Answer from the drawing. Dimensions are ordinates in mm from the lowest x, y and z of the part. Give positions to 0.01 mm unless a question says otherwise; leave off trailing zeros. Order: outer loops, then holes, each group sorted by start corner. A loop starts at its lowest first (then second) coordinate and runs counter-clockwise, first axis right, second up. Notation, with made-up numbers: (69.25, 32) - (115.25, 32) arc R19 ccw to (115.25, 69) - close; hole circle Ø4 at (37.5, 69.5). An arc over 180 degrees is marked (long way). Write each question's results on one line, items separated by ' | '.
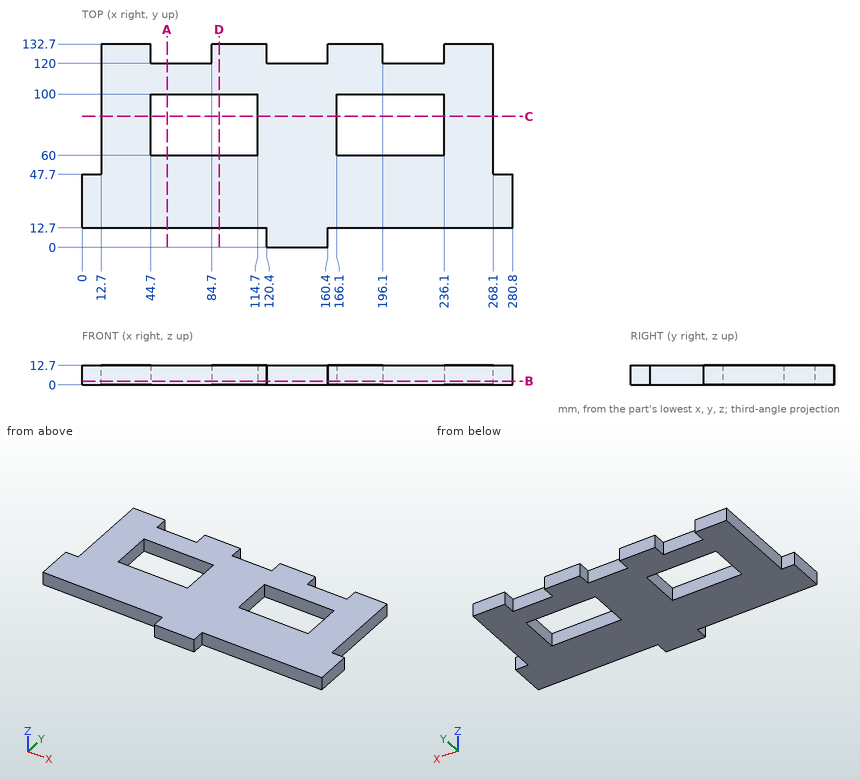
(1) Section A-A (x = 55.5) is taken. Give the vertices of the cut face in (y, z).
Conclusion:
outline: (12.7, 0) - (60, 0) - (60, 12.7) - (12.7, 12.7) - close; (100, 0) - (120, 0) - (120, 12.7) - (100, 12.7) - close
(2) Section B-B (z = 2.5) is taken. State how many separate pieces and enclosed holes the cut face has, plus the area to 3 significant figures.
Conclusion:
separate pieces: 1 | enclosed holes: 2 | area: 24,900 mm^2
(3) Consider probe 1 along X at (y, z) = (122, 6); probe 2 along X at (y, z) = (96.5, 9); probe 3 along Y at (x, z) = (93, 1.5). Determine where each line is inside the solid, lowest interval first. Write a range as [from, to].
Conclusion:
probe 1: [12.7, 44.7], [84.7, 120.4], [160.4, 196.1], [236.1, 268.1] | probe 2: [12.7, 44.7], [114.7, 166.1], [236.1, 268.1] | probe 3: [12.7, 60], [100, 132.7]
(4) Section D-D (x = 89.5) is taken. Give the vertices of the cut face in (y, z).
Conclusion:
outline: (12.7, 0) - (60, 0) - (60, 12.7) - (12.7, 12.7) - close; (100, 0) - (132.7, 0) - (132.7, 12.7) - (100, 12.7) - close
(5) Section C-C (y = 85.5) is taken. Give the vertices of the cut face in (x, z), plus the area to 3 significant figures.
Conclusion:
outline: (12.7, 0) - (44.7, 0) - (44.7, 12.7) - (12.7, 12.7) - close; (114.7, 0) - (166.1, 0) - (166.1, 12.7) - (114.7, 12.7) - close; (236.1, 0) - (268.1, 0) - (268.1, 12.7) - (236.1, 12.7) - close | area: 1,470 mm^2
(6) Each of these flat-tipped pins is pushed along its axis until it touches: pin 1 (3 mm diameter, centred on y = 111, z = 4, fed in from +X); pin 2 (4 mm diameter, centred on y = 127, z = 7.5, fed in from -X); pin 3 (6.5 mm diameter, centred on x = 56, z = 4, fed in from +Y). Where does it stop, or does it pass through?
Conclusion:
pin 1: x = 268.1 | pin 2: x = 12.7 | pin 3: y = 120
